Work out the finished part from the listing and answer in its coordinate system (mm). A direction names the side the tool comes from. Round coordinates to 2 decimals unless told otherwise and drop trailing zeros. Write each loop counter-clockwise with the first axis right and the second up, starting at its lowest first coordinate (ties: lowest second). Pieces come first, ordered by that corner, then holes. Notation, with made-up numbers: M 57.5,4.25 L 69.5,4.25 A9 cw 69.5,14.25 Z; hole C -4,12.5 d8. An arc over 180 degrees is marked long. Answer in a Markdown table with one row per item.
```python
from build123d import *

# Parameters (mm, degrees)
BOSS_EXTRUDE1_DEPTH      = 90
CUT_EXTRUDE_3_DEPTH      = 96.450944476
CUT_EXTRUDE_3_DEPTH_BACK = 96.450944476
SKETCH_1_R               = 1.75


with BuildPart() as part:
    # Sketch3 → Boss-Extrude1 (new body)
    with BuildSketch(Plane.XY):
        with BuildLine():
            ThreePointArc((28.391540767, 5.745528826), (28.540330522, 5.386318581), (28.899540767, 5.237528826))
            Line((28.899540767, 5.237528826), (29.981834767, 5.237528826))
            ThreePointArc((29.981834767, 5.237528826), (30.17623795, 5.276198023), (30.341045012, 5.386318581))
            Line((30.341045012, 5.386318581), (32.435619517, 7.480893087))
            ThreePointArc((32.435619517, 7.480893087), (33.154438301, 7.774195584), (33.870518646, 7.474269363))
            Line((33.870518646, 7.474269363), (36.110112773, 5.234675237))
            Line((36.110112773, 5.234675237), (39.091540767, 5.234675237))
            Line((39.091540767, 5.234675237), (41.08974786, 3.234676041))
            Line((41.08974786, 3.234676041), (41.084369139, -2.765323955))
            Line((41.084369139, -2.765323955), (45.091540767, -2.765323955))
            Line((45.091540767, -2.765323955), (45.091540767, 7.191225138))
            Line((45.091540767, 7.191225138), (41.088844083, 7.191225138))
            Line((41.088844083, 7.191225138), (38.591540767, 7.191225138))
            Line((38.591540767, 7.191225138), (38.591540767, 19.191225138))
            Line((38.591540767, 19.191225138), (41.091540767, 19.191225138))
            Line((41.091540767, 19.191225138), (45.091540767, 19.191225138))
            Line((45.091540767, 19.191225138), (45.091540767, 29.147775237))
            Line((45.091540767, 29.147775237), (41.091540767, 29.147775237))
            Line((41.091540767, 29.147775237), (41.091540767, 23.147775237))
            Line((41.091540767, 23.147775237), (39.091540767, 21.147775237))
            Line((39.091540767, 21.147775237), (36.112970002, 21.147775237))
            Line((36.112970002, 21.147775237), (33.873375875, 18.908181111))
            ThreePointArc((33.873375875, 18.908181111), (33.154687691, 18.609685261), (32.435619517, 18.907264564))
            Line((32.435619517, 18.907264564), (30.341045012, 21.00183907))
            ThreePointArc((30.341045012, 21.00183907), (30.17623795, 21.111959628), (29.981834767, 21.150628826))
            Line((29.981834767, 21.150628826), (28.899540767, 21.150628826))
            ThreePointArc((28.899540767, 21.150628826), (28.540330522, 21.00183907), (28.391540767, 20.642628826))
            Line((28.391540767, 20.642628826), (28.391540767, 5.745528826))
        make_face()
    extrude(amount=BOSS_EXTRUDE1_DEPTH)

    # Эскиз1 → Вырез-Вытянуть3 (cut, two sides: drawn at the far end of the back side and taken through both)
    with BuildSketch(Plane.ZY.offset(-41.091540767).offset(-CUT_EXTRUDE_3_DEPTH_BACK)):
        with Locations(Location((10, 0.026075116, 0), (0, 0, 270))):
            Circle(SKETCH_1_R)
        with Locations(Location((45, 0.026075116, 0), (0, 0, 270))):
            Circle(SKETCH_1_R)
        with Locations(Location((80, 0.026075116, 0), (0, 0, 270))):
            Circle(SKETCH_1_R)
        with Locations(Location((45, 26.147775237, 0), (0, 0, 270))):
            Circle(SKETCH_1_R)
        with Locations(Location((80, 26.147775237, 0), (0, 0, 270))):
            Circle(SKETCH_1_R)
        with Locations(Location((10, 26.147775237, 0), (0, 0, 270))):
            Circle(SKETCH_1_R)
    extrude(amount=CUT_EXTRUDE_3_DEPTH + CUT_EXTRUDE_3_DEPTH_BACK, mode=Mode.SUBTRACT)


solid = part.part
```
1. The part is cut by section D-D (z = 66). Determine the outline of the cut face in (x, y).
Calculated:
| item | result |
|---|---|
| outline | M 28.39,5.75 A0.51 ccw 28.9,5.24 L 29.98,5.24 A0.51 ccw 30.34,5.39 L 32.44,7.48 A1.02 cw 33.87,7.47 L 36.11,5.23 L 39.09,5.23 L 41.09,3.23 L 41.08,-2.77 L 45.09,-2.77 L 45.09,7.19 L 38.59,7.19 L 38.59,19.19 L 45.09,19.19 L 45.09,29.15 L 41.09,29.15 L 41.09,23.15 L 39.09,21.15 L 36.11,21.15 L 33.87,18.91 A1.02 cw 32.44,18.91 L 30.34,21 A0.51 ccw 29.98,21.15 L 28.9,21.15 A0.51 ccw 28.39,20.64 Z |
2. Consider line 1 along Y through (x, z) = (42.05, 80); line 2 along Y through (x, z) = (43.75, 76); line 3 along Y through (x, z) = (36.25, 35). Determine where each line is inside the solid, lowest interval first. Write a range as from..to.
Calculated:
| item | result |
|---|---|
| line 1 | y = -2.77..-1.72, 1.78..7.19, 19.19..24.4, 27.9..29.15 |
| line 2 | y = -2.77..7.19, 19.19..29.15 |
| line 3 | y = 5.23..21.15 |
3. The part is cut by section C-C (x = 40.25). Determine the outline of the cut face in (y, z), plus the area to 3 significant figures.
Calculated:
| item | result |
|---|---|
| outline | M 4.08,0 L 7.19,0 L 7.19,90 L 4.08,90 Z; M 19.19,0 L 22.31,0 L 22.31,90 L 19.19,90 Z |
| area | 561 mm² |
4. Given pin 1 (5 mm diameter, centred on x = 33.5, z = 55, fed in from +Y); pin 2 (0.9 mm diameter, centred on x = 37.5, z = 39.5, fed in from +Y); pin 3 (8 mm diameter, centred on x = 30.5, z = 69.5, fed in from -Y), each flat-ended and moving along its own axis, determine where each tip first touches the part or whether it passes through.
Calculated:
| item | result |
|---|---|
| pin 1 | stops at y = 21.03 |
| pin 2 | stops at y = 21.15 |
| pin 3 | stops at y = 5.24 |
5. The part is cut by section B-B (y = 1). Determine the outline of the cut face in (x, z).
Calculated:
| item | result |
|---|---|
| outline | M 41.09,0 L 45.09,0 L 45.09,8.55 L 41.09,8.55 Z; M 41.09,11.45 L 45.09,11.45 L 45.09,43.55 L 41.09,43.55 Z; M 41.09,46.45 L 45.09,46.45 L 45.09,78.55 L 41.09,78.55 Z; M 41.09,81.45 L 45.09,81.45 L 45.09,90 L 41.09,90 Z |
6. Determine the mould class of faces 1 (the flat face through (38, 21.148, 44)), 2 (the flat face through (42, 7.191, 44)), 3 (the flat face through (28.392, 13, 44)) for opening direction Y: released by +Y, released by -Y, zero draft, split by the parting line, or undercut.
Calculated:
| item | result |
|---|---|
| face 1 | released by +Y |
| face 2 | undercut |
| face 3 | zero draft |
7. A tool of negligible diameter and unlimited length cuts with its end or side. For faces 4 (the flat face through (43, -2.765, 44)), 5 (the flat face through (42, 19.191, 44)), 6 (the flat face through (35.009, 20.044, 44.37)), from which of +Z, -Z, +X, -X, +Y, -Y can it reach the whole face along a straight path? Write none if from no direction.
Calculated:
| item | result |
|---|---|
| face 4 | +Z, -Z, +X, -X, -Y |
| face 5 | +Z, -Z, +X |
| face 6 | +Z, -Z, +Y |
8. The part is cut by section A-A (z = 45). Count the separate pieces of the cut face and the enclosed holes in it, plus the area to 3 significant figures.
Calculated:
| item | result |
|---|---|
| separate pieces | 3 |
| enclosed holes | 0 |
| area | 211 mm² |
